Source: CAD feature listing. Evaluate the final solid. Frame: model axes, mm. Face numbers are marked on the shaded views. A direction names the side the tool comes from. Coordinates: 2 decimals unless noted, no trailing zeros. Order: outer loops, then holes, each group sorted by start corner. A loop starts at its lowest first (then second) coordinate and runs counter-clockwise, first axis right, second up.
Item 1: Section A-A on z = 29. Return the cut outline in (x, y).
Item 2: Section D-D on z = 7. Return the cut outline in (x, y), then the cut area to 3 significant figures.
Item 3: Section B-B on z = 17. Return the cut outline in (x, y), then the cut area to 3 significant figures.
Item 4: Contact query for flat-ended pins moving along their axis: P1, Ø2.5, axis at x = 2, z = 25, coming from the -Y side; P2, Ø1.9, axis at y = 2.5, z = 16, coming from the -X side; P3, Ø3, axis at y = 12.5, z = 14, coming from the -X side; P4, Ø10, axis at x = 17.5, z = 25.5, coming from the +Y side. Output: stop coordinate, or through.
Item 5: Ray query, line 1 (Y direction, x = 6, z = 16.5); line 2 (Z direction, x = 24, y = 6); line 3 (X direction, y = 2, z = 15.5). Return the intervals inside material, ascending.
Item 6: Reachability of the marked faces 1, 2 and 3 from +Z, -Z, +X, -X, +Y, -Y: full face, straight path, thin tool, end or side. Return the list, or none.
Item 7: Section C-C on x = 17.5. Return the cut outline in (y, z) (1 decimal), then the cut area to 3 significant figures.
Item 8: Mould query, pull axis X, two halves, no side actions, for the marked faces 4, 5, 6 and 7. Classes: released by +X, released by -X, zero draft, split by the parting line, or undercut.
Autodesk Inventor part; units mm, degrees
ref_plane "YZ Plane" through (0, 0, 0) normal (1, 0, 0) x (0, 1, 0)
ref_plane "XZ Plane" through (0, 0, 0) normal (0, 1, 0) x (-1, 0, 0)
ref_plane "XY Plane" through (0, 0, 0) normal (0, 0, 1) x (1, 0, 0)
sketch "Sketch1" plane through (0, 0, 0) normal (0, 0, 1) x (1, 0, 0)
  line L0 (-6.3366, 6.9163) -> (21.6034, 6.9163)
  line L1 (21.6034, 6.9163) -> (21.6034, -8.3237)
  line L2 (21.6034, -8.3237) -> (-6.3366, -8.3237)
  line L3 (-6.3366, -8.3237) -> (-6.3366, 6.9163)
  point P0 (0, 0)
  dimension "d0" = 27.94
  dimension "d1" = 15.24
extrude "Extrusion1" add sketch "Sketch1" along normal blind 7.62
sketch "Sketch2" plane through (0, 0, 7.62) normal (0, 0, 1) x (1, 0, 0)
  line L0 (-6.3366, 6.9163) -> (-6.3366, -8.3237)
  line L1 (21.6034, -8.3237) -> (21.6034, 6.9163)
  line L2 (21.6034, -0.052) -> (21.6034, 2.361)
  line L3 (-6.3366, 2.361) -> (-6.3366, -0.052)
  line L4 (21.6034, 6.9163) -> (-6.3366, 6.9163)
  line L5 (-6.3366, -8.3237) -> (21.6034, -8.3237)
  line L6 (0.9631, 2.361) -> (-0.2406, 2.361)
  line L7 (-0.2406, -0.052) -> (0.9631, -0.052)
  line L8 (-0.2406, -0.052) -> (-0.2406, 2.361)
  line L9 (-0.2406, -0.052) -> (3.0821, -0.052)
  line L10 (3.0821, -0.052) -> (3.0821, 2.361)
  line L11 (3.0821, 2.361) -> (-0.2406, 2.361)
  line L12 (-0.2406, 2.361) -> (-0.2406, -0.052)
  line L13 (14.3038, 2.361) -> (15.5074, 2.361)
  line L14 (15.5074, -0.052) -> (14.3038, -0.052)
  line L15 (15.5074, -0.052) -> (15.5074, 2.361)
  line L16 (15.5074, -0.052) -> (12.1847, -0.052)
  line L17 (12.1847, -0.052) -> (12.1847, 2.361)
  line L18 (12.1847, 2.361) -> (15.5074, 2.361)
  line L19 (15.5074, 2.361) -> (15.5074, -0.052)
  line L20 (-6.3366, -0.7037) -> (21.6034, -0.7037)
  line L21 (-6.3366, 2.361) -> (21.6034, 2.361)
  line L22 (21.6034, 2.361) -> (21.6034, -0.052)
  line L23 (21.6034, -0.052) -> (-6.3366, -0.052)
  line L24 (-6.3366, -0.052) -> (-6.3366, 2.361)
  point P0 (0, 0)
  point P1 (-0.2406, 1.1545)
  point P2 (15.2669, -0.3643)
  point P3 (15.5074, 1.1545)
  point P4 (15.5074, -0.052)
  point P5 (21.6034, -0.052)
  point P6 (15.5074, 2.361)
  point P7 (-6.3366, -0.052)
  point P8 (-0.2406, -0.052)
  point P9 (-0.2406, 2.361)
  point P10 (-6.3366, 2.361)
  point P11 (3.0821, -0.052)
  point P12 (12.1847, -0.052)
  point P13 (12.1847, 2.361)
  point P14 (3.0821, 2.361)
  dimension "d6" = 6.096
extrude "Extrusion2" add sketch "Sketch2" along normal blind 8.7376 contours L6 L11 L10 L9 L7 L8 | L15 L14 L16 L17 L18 L13
sketch "Sketch3" plane through (-0.2406, 2.361, 7.62) normal (0, 1, 0) x (1, 0, 0)
  line L0 (3.3227, -8.7376) -> (0, -8.7376)
  line L1 (-6.096, 7.62) -> (21.844, 7.62)
  line L2 (3.3227, -11.3552) -> (3.3227, -8.7376)
  line L3 (12.4253, -11.3552) -> (12.4253, -8.7376)
  line L4 (17.2091, -8.255) -> (17.2091, -15.2732)
  line L5 (17.2091, -15.2732) -> (14.9854, -19.057)
  line L6 (14.9854, -19.057) -> (12.4253, -19.057)
  line L7 (12.4253, -19.057) -> (12.4253, -8.7376)
  line L8 (7.874, 7.62) -> (7.874, -24.8322)
  line L9 (3.3227, -11.3552) -> (3.3227, -8.7376)
  line L10 (-1.4611, -8.255) -> (-1.4611, -15.2732)
  line L11 (-1.4611, -15.2732) -> (0.7626, -19.057)
  line L12 (0.7626, -19.057) -> (3.3227, -19.057)
  line L13 (3.3227, -19.057) -> (3.3227, -8.7376)
  line L14 (17.2091, -8.255) -> (12.4253, -8.255)
  line L15 (12.4253, 0) -> (12.4253, -8.7376)
  line L16 (12.4253, -8.255) -> (12.4253, -8.7376)
  line L17 (-1.4611, -8.255) -> (3.3227, -8.255)
  line L18 (3.3227, 0) -> (3.3227, -8.7376)
  line L19 (3.3227, -8.255) -> (3.3227, -8.7376)
  point P0 (0.2406, 7.62)
extrude "Extrusion4" add sketch "Sketch2" along normal blind 25.4 contours L6 L11 L10 L9 L7 L8 | L15 L14 L16 L17 L18 L13
sketch "Sketch4" plane through (-6.3366, 6.9163, 0) normal (0, 1, 0) x (1, 0, 0)
  point P0 (6.3366, 0)
sketch "Sketch5" plane through (0, 0, 7.62) normal (0, 0, 1) x (1, 0, 0)
  line L0 (21.6034, 6.9163) -> (-6.3366, 6.9163)
  line L1 (-6.3366, 15.6735) -> (21.6034, 15.6735)
  line L2 (21.6034, 15.6735) -> (21.6034, 6.9163)
  line L3 (21.6034, 6.9163) -> (-6.3366, 6.9163)
  line L4 (-6.3366, 6.9163) -> (-6.3366, 15.6735)
  point P0 (0, 0)
extrude "Extrusion5" add sketch "Sketch5" along normal blind 17.145 and the other way blind 7.62
extrude "Extrusion6" cut sketch "Sketch2" against normal blind 25.4 contours L20 L1 L5 L0
extrude "Extrusion7" add sketch "Sketch2" along normal blind 4.7625 contours L21 L8 L23 L0 | L1 L23 L15 L21 | L21 L17 L23 L10
extrude "Extrusion8" add sketch "Sketch3" against normal up to surface (2.413 mm away)
sketch "Sketch6" plane through (-6.3366, -0.052, 7.62) normal (0, -1, 0) x (1, 0, 0)
  line L0 (27.94, 0) -> (27.94, 4.7625)
  line L1 (21.844, 4.7625) -> (21.844, 8.255)
  line L2 (27.94, 0) -> (21.844, 0)
  line L3 (21.844, 0) -> (21.844, 4.7625)
  line L4 (21.844, 4.7625) -> (27.94, 4.7625)
  line L5 (27.94, 4.7625) -> (27.94, 0)
  line L6 (18.5213, 4.7625) -> (18.5213, 25.4)
  line L7 (18.5213, 4.7625) -> (9.4187, 4.7625)
  line L8 (9.4187, 4.7625) -> (9.4187, 0)
  line L9 (9.4187, 0) -> (18.5213, 0)
  line L10 (18.5213, 0) -> (18.5213, 4.7625)
  line L11 (6.096, 4.7625) -> (6.096, 8.255)
  line L12 (0, 0) -> (0, 4.7625)
  line L13 (6.096, 4.7625) -> (0, 4.7625)
  line L14 (0, 4.7625) -> (0, 0)
  line L15 (0, 0) -> (6.096, 0)
  line L16 (6.096, 0) -> (6.096, 4.7625)
  point P0 (6.3366, -7.62)
  point P1 (21.844, 8.7376)
  point P2 (18.5213, 19.057)
  point P3 (6.096, 8.7376)
extrude "Extrusion9" cut sketch "Sketch6" against normal up to surface (6.9683 mm away)
sketch "Sketch7" plane through (12.1847, -0.052, 7.62) normal (0, -1, 0) x (1, 0, 0)
  line L0 (3.3227, 17.7594) -> (4.7838, 15.2732)
  line L1 (3.3227, 17.7594) -> (2.3659, 19.3874)
  line L2 (2.3659, 19.3874) -> (2.3659, 25.4)
  line L3 (3.3227, 25.4) -> (0, 25.4)
  line L4 (3.3227, 17.7594) -> (3.3227, 25.4)
  line L5 (2.3659, 25.4) -> (3.3227, 25.4)
  line L6 (3.3227, 25.4) -> (3.3227, 17.7594)
  line L7 (-18.5213, -7.62) -> (9.4187, -7.62)
  line L8 (-12.4253, 17.7594) -> (-11.4685, 19.3874)
  line L9 (-11.4685, 19.3874) -> (-11.4685, 25.4)
  line L10 (-12.4253, 17.7594) -> (-12.4253, 25.4)
  line L11 (-11.4685, 25.4) -> (-12.4253, 25.4)
  line L12 (-12.4253, 25.4) -> (-12.4253, 17.7594)
  line L13 (-12.4253, 8.7376) -> (-13.8865, 8.255)
  line L14 (-9.1825, 8.7376) -> (-9.1026, 8.7376)
  line L15 (-9.1026, 0) -> (-9.1026, 25.4)
  line L16 (-10.6842, 5.3569) -> (-10.764, 0)
  line L17 (-9.1026, 0) -> (-12.4253, 0)
  line L18 (-9.1026, 0) -> (-9.1026, 8.7376)
  line L19 (-10.764, 0) -> (-9.1026, 0)
  line L20 (9.4187, -7.62) -> (-18.5213, -7.62)
  line L21 (-18.5213, 17.145) -> (9.4187, 17.145)
  line L22 (1.5816, 5.3569) -> (1.6613, 0)
  line L23 (1.6613, 0) -> (0, 0)
  line L24 (0, 0) -> (0, 8.7376)
  line L25 (-4.5513, -7.62) -> (-4.5513, 0)
  line L26 (-4.5513, 11.274) -> (-4.5513, 11.3382)
  line L27 (-9.1026, 8.7376) -> (-10.6842, 5.3569)
  line L28 (0, 8.7376) -> (1.5816, 5.3569)
  point P0 (-12.1847, -7.62)
extrude "Extrusion10" cut sketch "Sketch7" against normal up to surface (6.9683 mm away)
fillet "Fillet1" radius 3.175 4 edges at (0.7162, 1.1545, 33.02) (14.5507, 1.1545, 33.02) (16.9686, 1.1545, 22.8932) (-1.7017, 1.1545, 22.8932)
sketch "Sketch8" plane through (-0.2406, -0.052, 7.62) normal (0, -1, 0) x (1, 0, 0)
  arc A0 (-1.0234, 16.018) -> (-1.4611, 14.4093) centre (1.7139, 14.4093) ccw
  line L0 (-1.4611, 8.255) -> (-1.4611, 14.4093)
  line L1 (0, 0) -> (0, 8.255)
  line L2 (1.6613, 0) -> (0, 0)
  line L3 (1.6613, 0) -> (1.7411, 5.3569)
  line L4 (1.7411, 5.3569) -> (3.3227, 8.7376)
  line L5 (3.3227, 8.7376) -> (3.3227, 25.4)
  arc A1 (3.3227, 25.4) -> (0.9568, 22.3298) centre (4.1318, 22.3298) ccw
  line L6 (0.9568, 22.3298) -> (0.9568, 19.3874)
  line L7 (0.9568, 19.3874) -> (-1.0234, 16.018)
  arc A2 (17.2091, 14.4093) -> (16.7714, 16.018) centre (14.0341, 14.4093) ccw
  line L8 (16.7714, 16.018) -> (14.7912, 19.3874)
  line L9 (14.7912, 19.3874) -> (14.7912, 22.3298)
  arc A3 (14.7912, 22.3298) -> (12.4253, 25.4) centre (11.6162, 22.3298) ccw
  line L10 (12.4253, 8.7376) -> (12.4253, 25.4)
  line L11 (12.4253, 8.7376) -> (14.0069, 5.3569)
  line L12 (14.0069, 5.3569) -> (14.0867, 0)
  line L13 (15.748, 0) -> (14.0867, 0)
  line L14 (15.748, 0) -> (15.748, 8.255)
  line L15 (17.2091, 14.4093) -> (17.2091, 8.255)
  line L16 (17.2091, 8.255) -> (15.748, 8.255)
  line L17 (0, 8.255) -> (-1.4611, 8.255)
  point P0 (0.2406, -7.62)
extrude "Extrusion11" add sketch "Sketch8" against normal blind 3.81
sketch "Sketch9" plane through (0, 0, 7.62) normal (0, 0, 1) x (1, 0, 0)
  line L0 (9.6447, 0.3123) -> (5.6221, 0.3123)
  line L1 (5.6221, 0.3123) -> (5.6221, 4.1223)
  line L2 (5.6221, 4.1223) -> (9.6447, 4.1223)
  line L3 (9.6447, 4.1223) -> (9.6447, 0.3123)
  line L4 (12.1847, -0.052) -> (12.1847, 3.758)
  line L5 (3.0821, -0.052) -> (3.0821, 3.758)
  point P0 (0, 0)
  dimension "d30" = 2.54
  dimension "d31" = 2.54
extrude "Extrusion12" add sketch "Sketch9" along normal blind 18.0975
sketch "Sketch10" plane through (21.6034, 6.9163, 24.765) normal (1, 0, 0) x (0, 0, -1)
  line L0 (17.145, 0) -> (0, 0)
  line L1 (24.765, -7.62) -> (17.145, -7.62)
  line L2 (17.145, 0) -> (24.765, 0)
  line L3 (24.765, 0) -> (24.765, -7.62)
  line L4 (24.765, -7.62) -> (17.145, -7.62)
  line L5 (17.145, -7.62) -> (17.145, 0)
  point P0 (24.765, -6.9163)
extrude "Extrusion13" add sketch "Sketch10" along normal blind 6.1214 and the other way blind 34.0614
sketch "Sketch11" plane through (0, 0, 7.62) normal (0, 0, 1) x (1, 0, 0)
  line L0 (21.6034, 15.6735) -> (-6.3366, 15.6735)
  line L1 (9.6447, 0.3123) -> (5.6221, 0.3123)
  line L2 (-12.458, -0.7037) -> (-12.458, 6.9163)
  line L3 (-12.458, -0.7037) -> (27.7248, -0.7037)
  line L4 (-11.1046, -0.7037) -> (-12.458, -0.7037)
  line L5 (-12.458, -0.7037) -> (-12.458, 4.1961)
  line L6 (21.6034, -0.7037) -> (27.7131, -0.7037)
  line L7 (27.7131, -0.7037) -> (27.7131, 4.8182)
  line L8 (21.6034, 4.8182) -> (21.6034, -0.7037)
  line L9 (-6.3366, -0.7037) -> (-12.4462, -0.7037)
  line L10 (-12.4462, -0.7037) -> (-12.4462, 4.8182)
  line L11 (-6.3366, 4.8182) -> (-6.3366, -0.7037)
  line L12 (21.6034, 6.9163) -> (27.7248, 6.9163)
  line L13 (7.6334, 0.3123) -> (7.6334, -0.7037)
  line L14 (-12.4462, 3.7917) -> (-8.3234, 3.7917)
  line L15 (-8.3234, 3.7917) -> (-8.3234, -0.7037)
  line L16 (27.7248, -0.7037) -> (27.7248, 6.9163)
  line L17 (27.7248, -0.7037) -> (-12.458, -0.7037)
  line L18 (26.3715, -0.7037) -> (27.7248, -0.7037)
  line L19 (27.7248, -0.7037) -> (27.7248, 4.1961)
  line L20 (21.6034, -0.7037) -> (27.7131, -0.7037)
  line L21 (27.7131, -0.7037) -> (27.7131, 4.8182)
  line L22 (27.7131, 3.7917) -> (23.5902, 3.7917)
  line L23 (23.5902, 3.7917) -> (23.5902, -0.7037)
  point P0 (0, 0)
  point P1 (22.941, 6.9163)
  point P2 (-7.6742, 6.9163)
  point P3 (-7.6742, 3.7917)
  point P4 (-8.3234, -0.7037)
  point P5 (23.5902, -0.7037)
extrude "Extrusion15" add sketch "Sketch11" along normal blind 14.2875
properties part number "Attachment7"
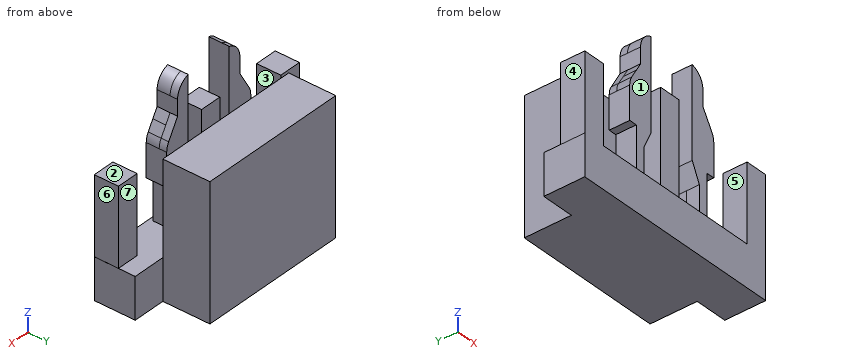
Answer list:
1. outline: (0.72, -0.05) - (3.08, -0.05) - (3.08, 3.76) - (0.72, 3.76) - close; (12.18, -0.05) - (14.55, -0.05) - (14.55, 3.76) - (12.18, 3.76) - close
2. outline: (-12.46, -0.7) - (27.72, -0.7) - (27.72, 6.92) - (21.6, 6.92) - (21.6, 15.67) - (-6.34, 15.67) - (-6.34, 6.92) - (-12.46, 6.92) - close
2. area: 551 mm2
3. outline: (-12.45, -0.7) - (-8.32, -0.7) - (-8.32, 3.79) - (-12.45, 3.79) - close; (-6.34, 6.92) - (21.6, 6.92) - (21.6, 15.67) - (-6.34, 15.67) - close; (-1.7, -0.05) - (3.08, -0.05) - (3.08, 3.76) - (-1.7, 3.76) - close; (5.62, 0.31) - (9.64, 0.31) - (9.64, 4.12) - (5.62, 4.12) - close; (12.18, -0.05) - (16.97, -0.05) - (16.97, 3.76) - (12.18, 3.76) - close; (23.59, -0.7) - (27.71, -0.7) - (27.71, 3.79) - (23.59, 3.79) - close
3. area: 334 mm2
4. P1: stops at y = -0.05
4. P2: stops at x = -12.45
4. P3: stops at x = -6.34
4. P4: stops at y = 15.67
5. line 1: y = 0.31 to 4.12, 6.92 to 15.67
5. line 2: z = 0 to 7.62
5. line 3: x = -12.45 to -8.32, -0.24 to 2.68, 5.62 to 9.64, 12.59 to 15.51, 23.59 to 27.71
6. face 1: +Z, -Y
6. face 2: +Z, +X, +Y, -Y
6. face 3: +Z, +Y, -Y
7. outline: (-0.7, 0) - (15.7, 0) - (15.7, 24.8) - (6.9, 24.8) - (6.9, 7.6) - (-0.7, 7.6) - close
7. area: 275 mm2
8. face 4: released by -X
8. face 5: undercut
8. face 6: released by +X
8. face 7: zero draft
